The listing builds one solid part. Answer for the finished solid, in the listing's coordinates (mm). Give positions to 0.01 mm unless a question says otherwise; leave off trailing zeros. Order: outer loops, then holes, each group sorted by start corner. A loop starts at its lowest first (then second) coordinate and runs counter-clockwise, first axis right, second up. Notation, with made-up numbers: (-27.5, 77) - (1.5, 77) arc R27 cw to (1.5, 103) - close; hole circle Ø9 at (19, 29). An arc over 180 degrees is marked (long way). Write each question's results on one line, items separated by ' | '. Start each with the question number.
1. Section A-A (y = -1.3) is taken. Give the vertices of the cut face in (x, z).
2. Section B-B (x = -12.5) is taken. Give the vertices of the cut face in (y, z), and give its area (3 significant figures).
3. Section C-C (z = -10.5) is taken. Give the vertices of the cut face in (x, y).
4. Find the intervals of material crossed by L1, parallel to X at y = -1.2, z = 18.5; L2, parallel to Z at x = -13, y = -3.3; L3, parallel to Z at x = 83.5, y = -1.7, in increasing order.
from build123d import *

# Parameters (mm, degrees)
F1_DEPTH = 4.7625


with BuildPart() as f1:
    # F0 (on Front) → F1 (new body)
    with BuildSketch(Plane.XZ):
        with BuildLine():
            Line((-44.46612, 20.617304), (-65.10362, 20.617304))
            Line((-65.10362, 20.617304), (-65.10362, -0.020196))
            Line((-65.10362, -0.020196), (-33.365841, -21.178716))
            ThreePointArc((-33.365841, -21.178716), (-31.683624, -21.972731), (-29.843495, -22.245196))
            Line((-29.843495, -22.245196), (11.794531, -22.245196))
            ThreePointArc((11.794531, -22.245196), (12.675284, -22.183819), (13.53901, -22.000873))
            Line((13.53901, -22.000873), (90.47138, -0.020196))
            Line((90.47138, -0.020196), (90.47138, 20.617304))
            Line((90.47138, 20.617304), (69.83388, 20.617304))
            Line((69.83388, 20.617304), (69.83388, 15.854804))
            Line((69.83388, 15.854804), (-44.46612, 15.854804))
            Line((-44.46612, 15.854804), (-44.46612, 20.617304))
        make_face()
    extrude(amount=F1_DEPTH)


solid = f1.part
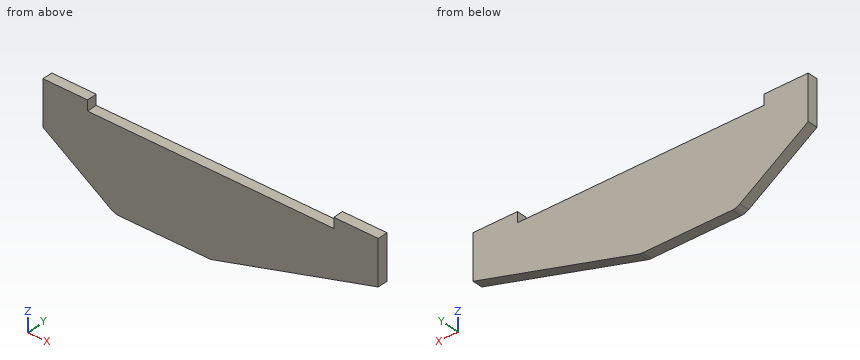
Reported:
1) outline: (-65.1, -0.02) - (-33.37, -21.18) arc R6.35 ccw to (-29.84, -22.25) - (11.79, -22.25) arc R6.35 ccw to (13.54, -22) - (90.47, -0.02) - (90.47, 20.62) - (69.83, 20.62) - (69.83, 15.85) - (-44.47, 15.85) - (-44.47, 20.62) - (-65.1, 20.62) - close
2) outline: (-4.76, -22.25) - (0, -22.25) - (0, 15.85) - (-4.76, 15.85) - close | area: 181 mm²
3) outline: (-49.38, -4.76) - (53.79, -4.76) - (53.79, 0) - (-49.38, 0) - close
4) L1: -65.1 to -44.47, 69.83 to 90.47 | L2: -22.25 to 15.85 | L3: -2.01 to 20.62
